Build history of the part. All positions in model axes, mm. Face numbers are marked on the shaded views. A direction names the side the tool comes from. Round coordinates to 2 decimals unless told otherwise and drop trailing zeros. Loops run counter-clockwise (first coordinate to the right, second up) from the corner with the lowest first, then second, coordinate; pieces in that order, holes last. Notation, with made-up numbers: (19.25, -13.75) - (60.25, -13.75) arc R32 cw to (60.25, 17.25) - close; hole circle Ø9 at (4, 18). An arc over 180 degrees is marked (long way). Use one line per item in the form item = value. Start each with the question number.
Q1. 3-axis set-ups, long thin cutter, end or side, ignore diameter. For the marked faces 1 and 2: which of +Z, -Z, +X, -X, +Y, -Y reach the whole face in a straight line?
Q2. Mould opens along X. For the marked faces 3, 4 and 5 say: released by +X, released by -X, zero draft, split by the parting line, or undercut.
Q3. Saw through at D-D (y = 11.5). Give the cut face in (x, z) (3 decimals), then the cut area to 3 significant figures.
Q4. Saw through at C-C (y = 6.5). Give the cut face in (x, z), then the cut area to 3 significant figures.
Q5. Pin check, flat tips, straight feed: pin 1 (7 mm diameter, centred on x = 10, y = 5.76, fed in from -Z); pin 2 (9 mm diameter, centred on x = 10, z = 18.925, fed in from -Y); pin 3 (4 mm diameter, centred on x = 13, y = 3, fed in from +Z). Stop position of each tip, or through.
Q6. Saw through at B-B (z = 17.25). Give the cut face in (x, y).
Q7. Saw through at A-A (x = 10). Give the cut face in (y, z).
Q8. Drill centre lines: line 1 (Z direction, x = 10, y = 11.85); line 2 (Y direction, x = 10, z = 2.4); line 3 (Z direction, x = 12.5, y = 7.25). Where is each one in solid material? Low to high.
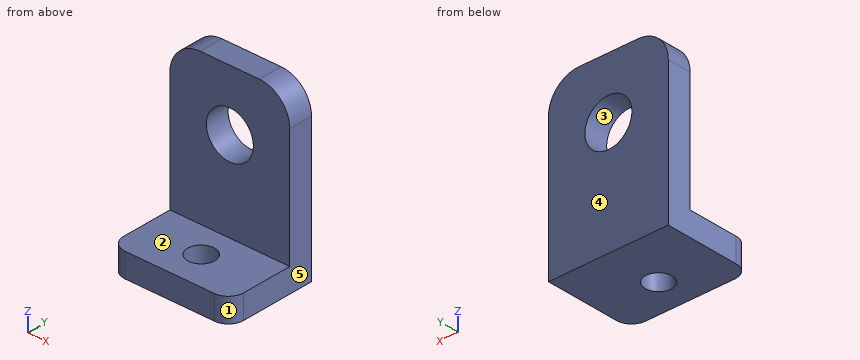
```python
from build123d import *

# Parameters (mm, degrees)
F0_W     = 20
F0_H     = 15
F1_DEPTH = 4
F2_W     = 20
F2_H     = 4
F3_DEPTH = 25
F4_R     = 2.25
F5_DEPTH = 25.4
F6_R     = 3.925
F7_DEPTH = 25.4
F8_R     = 2.54
F9_R     = 5.08


with BuildPart() as f1:
    # F0 (on Top) → F1 (new body)
    with BuildSketch(Plane.XY):
        with Locations((10, 7.5)):
            Rectangle(F0_W, F0_H)
    extrude(amount=F1_DEPTH)

    # F2 (on face) → F3 (join)
    with BuildSketch(Plane.XY.offset(4)):
        with Locations((10, 13)):
            Rectangle(F2_W, F2_H)
    extrude(amount=F3_DEPTH)

    # F4 (on face) → F5 (cut)
    with BuildSketch(Plane.XY.offset(4)):
        with Locations((10, 5.760205)):
            Circle(F4_R)
    extrude(amount=-F5_DEPTH, mode=Mode.SUBTRACT)

    # F6 (on face) → F7 (cut)
    with BuildSketch(Plane(origin=(0, 15, 0), x_dir=(-1, 0, 0), z_dir=(0, 1, 0))):
        with Locations((-10, 18.925)):
            Circle(F6_R)
    extrude(amount=-F7_DEPTH, mode=Mode.SUBTRACT)

    # F8
    f8_edges = [f1.edges().sort_by_distance(p)[0] for p in [
        (20, 0, 2),
        (0, 0, 2),
    ]]
    fillet(f8_edges, radius=F8_R)

    # F9
    f9_edges = [f1.edges().sort_by_distance(p)[0] for p in [
        (20, 13, 29),
        (0, 13, 29),
    ]]
    fillet(f9_edges, radius=F9_R)


solid = f1.part
```
Report:
q1.face_1 = +Z, -Z, +X, -Y
q1.face_2 = +Z, +X, -X, -Y
q2.face_3 = undercut
q2.face_4 = zero draft
q2.face_5 = released by +X
q3.outline = (0, 0) - (20, 0) - (20, 23.92) arc R5.08 ccw to (14.92, 29) - (5.08, 29) arc R5.08 ccw to (0, 23.92) - close; hole circle Ø7.85 at (10, 18.925)
q3.area = 521 mm²
q4.outline = (0, 0) - (7.88, 0) - (7.88, 4) - (0, 4) - close; (12.12, 0) - (20, 0) - (20, 4) - (12.12, 4) - close
q4.area = 63.0 mm²
q5.pin_1 = 0
q5.pin_2 = 11
q5.pin_3 = 4
q6.outline = (0, 11) - (6.45, 11) - (6.45, 15) - (0, 15) - close; (13.55, 11) - (20, 11) - (20, 15) - (13.55, 15) - close
q7.outline = (0, 0) - (3.51, 0) - (3.51, 4) - (0, 4) - close; (8.01, 0) - (15, 0) - (15, 15) - (11, 15) - (11, 4) - (8.01, 4) - close; (11, 22.85) - (15, 22.85) - (15, 29) - (11, 29) - close
q8.line_1 = 0 to 15, 22.85 to 29
q8.line_2 = 0 to 3.51, 8.01 to 15
q8.line_3 = 0 to 4
